Read the model definition and answer for the solid it produces. Units are mm, in the model's axes. Coordinates: 2 decimals unless noted, no trailing zeros. Write each loop counter-clockwise with the first axis right and the second up, starting at its lowest first coordinate (ties: lowest second). Pieces come first, ordered by that corner, then holes. Notation, with made-up numbers: M 70,64 L 94,64 A28 ccw 94,101 Z; hole C 60,78 d4. An arc over 180 degrees is marked long. Use a Markdown table: item, result. Add a question column.
from build123d import *

# Parameters (mm, degrees)
BOSS_EXTRUDE1_DEPTH = 3
FILLET1_R           = 10
FILLET2_R           = 0.2


with BuildPart() as part:
    # Sketch1 → Boss-Extrude1 (new body)
    with BuildSketch(Plane.XY):
        with BuildLine():
            Line((42.358686368, 22.000000982), (49.772401671, 22.000000982))
            add(Edge.make_bspline(
                [(49.772401671, 22.000000982), (49.840272704, 22.116351885), (50.1551903, 22.666226688), (50.950894785, 24.093636109), (51.94551412, 25.26324692), (52.886288967, 25.69272444)],
                knots=[0.181427978, 0.181427978, 0.181427978, 0.181427978, 0.24891213, 0.498932816, 1, 1, 1, 1], degree=3))
            add(Edge.make_bspline(
                [(52.886288967, 25.69272444), (54.227657261, 26.21198845), (56.978395025, 25.93722039), (59.747728448, 25.781572291), (61.056734627, 26.357306144)],
                knots=[0, 0, 0, 0, 0.501451854, 1, 1, 1, 1], degree=3))
            add(Edge.make_bspline(
                [(61.056734627, 26.357306144), (61.938277564, 26.747818697), (62.640002805, 27.412818263)],
                knots=[0, 0, 0, 1, 1, 1], degree=2))
            add(Edge.make_bspline(
                [(62.640002805, 27.412818263), (64.422298684, 32.447991264), (67.947295887, 42.570792519), (71.63632388, 52.63498927), (73.468775284, 57.690378858)],
                knots=[0, 0, 0, 0, 0.498322561, 1, 1, 1, 1], degree=3))
            add(Edge.make_bspline(
                [(73.468775284, 57.690378858), (73.65195235, 58.18791707), (73.947138477, 59.154492844), (73.494544705, 60.065888317), (73.136484432, 60.270519593)],
                knots=[0, 0, 0, 0, 0.581397084, 1, 1, 1, 1], degree=3))
            add(Edge.make_bspline(
                [(73.136484432, 60.270519593), (71.219763549, 60.304316664), (67.414772669, 60.120408261), (63.601790951, 60.225145139), (61.721316332, 60.4659848)],
                knots=[0, 0, 0, 0, 0.503014916, 1, 1, 1, 1], degree=3))
            add(Edge.make_bspline(
                [(61.721316332, 60.4659848), (61.953278841, 61.133157294), (62.437522451, 62.08211133), (63.355516567, 63.142847502), (64.128800308, 63.865372538), (65.076762001, 64.419081128), (66.503780011, 65.101780751), (67.695837691, 65.416597624), (68.523505542, 65.548080187)],
                knots=[0, 0, 0, 0, 0.237267367, 0.352023708, 0.469658656, 0.590380818, 0.718477308, 1, 1, 1, 1], degree=3))
            add(Edge.make_bspline(
                [(68.523505542, 65.548080187), (71.635771568, 65.94651733), (75.497539161, 66.798521287), (80.119338716, 67.878335493), (83.19923981, 68.360811237), (85.492331103, 68.508361677), (86.994967622, 68.519151336)],
                knots=[0, 0, 0, 0, 0.501477793, 0.632810111, 0.759518477, 1, 1, 1, 1], degree=3))
            add(Edge.make_bspline(
                [(86.994967622, 68.519151336), (87.203463843, 68.519151336), (87.796374971, 68.519151336), (88.3892861, 68.519151336), (88.773701007, 68.519151336)],
                knots=[0, 0, 0, 0, 0.351648352, 1, 1, 1, 1], degree=3))
            Line((88.773701007, 68.519151336), (74.524287403, 27.881934761))
            add(Edge.make_bspline(
                [(74.524287403, 27.881934761), (74.471104748, 27.682138266), (74.802744483, 27.172445206), (75.080434831, 26.689662332), (75.384334314, 26.415945707)],
                knots=[0, 0, 0, 0, 0.324502414, 1, 1, 1, 1], degree=3))
            Line((75.384334314, 26.415945707), (83.554779975, 26.103201375))
            add(Edge.make_bspline(
                [(83.554779975, 26.103201375), (82.959840411, 25.089982249), (82.414680301, 23.767742871), (81.574001976, 22.395101634), (81.262536262, 22.101391942), (81.138983475, 22.000000982)],
                knots=[0, 0, 0, 0, 0.504343167, 0.619768133, 0.688442197, 0.688442197, 0.688442197, 0.688442197], degree=3))
            Line((81.138983475, 22.000000982), (100, 22.000000982))
            Line((100, 22.000000982), (100, 0))
            Line((100, 0), (80, 0))
            Line((80, 0), (80, -3))
            Line((80, -3), (20, -3))
            Line((20, -3), (20, 0))
            Line((20, 0), (0, 0))
            Line((0, 0), (0, 22.000000982))
            Line((0, 22.000000982), (10.992104564, 22.000000982))
            add(Edge.make_bspline(
                [(10.992104564, 22.000000982), (11.059975596, 22.116351885), (11.374893193, 22.666226688), (12.170597678, 24.093636109), (13.165217013, 25.26324692), (14.105991859, 25.69272444)],
                knots=[0.181427978, 0.181427978, 0.181427978, 0.181427978, 0.24891213, 0.498932816, 1, 1, 1, 1], degree=3))
            add(Edge.make_bspline(
                [(14.105991859, 25.69272444), (15.447360154, 26.21198845), (18.198097918, 25.93722039), (20.967431341, 25.781572291), (22.27643752, 26.357306144)],
                knots=[0, 0, 0, 0, 0.501451854, 1, 1, 1, 1], degree=3))
            add(Edge.make_bspline(
                [(22.27643752, 26.357306144), (23.157980457, 26.747818697), (23.859705698, 27.412818263)],
                knots=[0, 0, 0, 1, 1, 1], degree=2))
            add(Edge.make_bspline(
                [(23.859705698, 27.412818263), (25.642001577, 32.447991264), (29.16699878, 42.570792519), (32.856026773, 52.63498927), (34.688478177, 57.690378858)],
                knots=[0, 0, 0, 0, 0.498322561, 1, 1, 1, 1], degree=3))
            add(Edge.make_bspline(
                [(34.688478177, 57.690378858), (34.871655243, 58.18791707), (35.16684137, 59.154492844), (34.714247598, 60.065888317), (34.356187325, 60.270519593)],
                knots=[0, 0, 0, 0, 0.581397084, 1, 1, 1, 1], degree=3))
            add(Edge.make_bspline(
                [(34.356187325, 60.270519593), (32.439466442, 60.304316664), (28.634475562, 60.120408261), (24.821493844, 60.225145139), (22.941019225, 60.4659848)],
                knots=[0, 0, 0, 0, 0.503014916, 1, 1, 1, 1], degree=3))
            add(Edge.make_bspline(
                [(22.941019225, 60.4659848), (23.172981734, 61.133157294), (23.657225344, 62.08211133), (24.57521946, 63.142847502), (25.348503201, 63.865372538), (26.296464893, 64.419081128), (27.723482904, 65.101780751), (28.915540584, 65.416597624), (29.743208435, 65.548080187)],
                knots=[0, 0, 0, 0, 0.237267367, 0.352023708, 0.469658656, 0.590380818, 0.718477308, 1, 1, 1, 1], degree=3))
            add(Edge.make_bspline(
                [(29.743208435, 65.548080187), (32.85547446, 65.94651733), (36.717242054, 66.798521287), (41.339041609, 67.878335493), (44.418942703, 68.360811237), (46.712033996, 68.508361677), (48.214670515, 68.519151336)],
                knots=[0, 0, 0, 0, 0.501477793, 0.632810111, 0.759518477, 1, 1, 1, 1], degree=3))
            add(Edge.make_bspline(
                [(48.214670515, 68.519151336), (48.423166736, 68.519151336), (49.016077864, 68.519151336), (49.608988993, 68.519151336), (49.9934039, 68.519151336)],
                knots=[0, 0, 0, 0, 0.351648352, 1, 1, 1, 1], degree=3))
            Line((49.9934039, 68.519151336), (35.743990296, 27.881934761))
            add(Edge.make_bspline(
                [(35.743990296, 27.881934761), (35.690807641, 27.682138266), (36.022447376, 27.172445206), (36.300137724, 26.689662332), (36.604037207, 26.415945707)],
                knots=[0, 0, 0, 0, 0.324502414, 1, 1, 1, 1], degree=3))
            Line((36.604037207, 26.415945707), (44.774482868, 26.103201375))
            add(Edge.make_bspline(
                [(44.774482868, 26.103201375), (44.179543303, 25.089982249), (43.634383194, 23.767742871), (42.793704869, 22.395101634), (42.482239154, 22.101391942), (42.358686368, 22.000000982)],
                knots=[0, 0, 0, 0, 0.504343167, 0.619768133, 0.688442197, 0.688442197, 0.688442197, 0.688442197], degree=3))
        make_face()
    extrude(amount=BOSS_EXTRUDE1_DEPTH)

    # Fillet1
    fillet1_edges = [part.edges().sort_by_distance(p)[0] for p in [
        (100, 22.000000982, 1.5),
        (0, 22.000000982, 1.5),
    ]]
    fillet(fillet1_edges, radius=FILLET1_R)

    # Fillet2
    fillet2_edges = [part.edges().sort_by_distance(p)[0] for p in [
        (49.772401671, 22.000000982, 1.5),
        (81.138983475, 22.000000982, 1.5),
        (42.358686368, 22.000000982, 1.5),
        (10.992104564, 22.000000982, 1.5),
    ]]
    fillet(fillet2_edges, radius=FILLET2_R)


solid = part.part
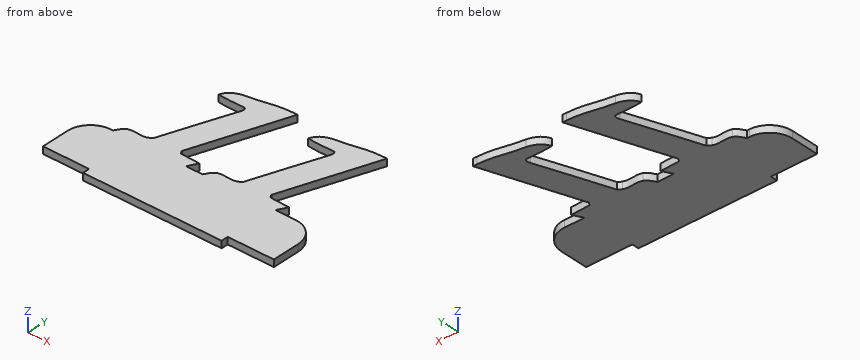
Item 1: Each of these flat-tipped pins is pushed along its axis until it touches: pin 1 (1.5 mm diameter, centred on x = 81, y = 58, fed in from -Z); pin 2 (0.9 mm diameter, centred on x = 89.5, z = 1.5, fed in from -Y); pin 3 (0.9 mm diameter, centred on x = 85, z = 2, fed in from +Y). Where does it stop, or does it pass through?
Item 2: Consider probe 1 along X at (y, z) = (29, 1.95); probe 2 along X at (y, z) = (37, 0.55); probe 3 along Y at (x, z) = (23.5, 1). Determine where each line is inside the solid, lowest interval first.
Item 3: Find section A-A on x = 7. Give the vertices of the cut face in (y, z), then the cut area to 3 significant figures.
Geometry says:
| question | item | result |
|---|---|---|
| 1 | pin 1 | stops at z = 0 |
| 1 | pin 2 | stops at y = 0 |
| 1 | pin 3 | stops at y = 68.48 |
| 2 | probe 1 | x = 24.42 to 36.14, 63.2 to 74.92 |
| 2 | probe 2 | x = 27.24 to 38.94, 66.02 to 77.72 |
| 2 | probe 3 | y = -3 to 27.1, 60.4 to 61.7 |
| 3 | outline | M 0,0 L 21.54,0 L 21.54,3 L 0,3 Z |
| 3 | area | 64.6 mm2 |
